from build123d import *

# Parameters (mm, degrees)
SKETCH1_R           = 13.155
BOSS_EXTRUDE1_DEPTH = 10
CHAMFER4_SIZE       = 10


with BuildPart() as part:
    # Sketch1 → Boss-Extrude1 (new body)
    with BuildSketch(Plane(origin=(0, 0, 0), x_dir=(1, 0, 0), z_dir=(0, 1, 0))):
        Polygon((0, 0), (37.5, 64.951905284), (0, 129.903810568), (64.951905284, 92.403810568), (129.903810568, 129.903810568), (92.403810568, 64.951905284), (129.903810568, 0), (64.951905284, 37.5), align=None)
        with Locations(Location((64.951905284, 64.951905284, 0), (0, 0, 270))):
            Circle(SKETCH1_R, mode=Mode.SUBTRACT)
    extrude(amount=BOSS_EXTRUDE1_DEPTH)

    # Chamfer4
    # the kernel refuses this chamfer: 10 mm, written as the material it takes off along each edge
    with BuildSketch(Plane(origin=(64.951905284, 10, -64.951905284), x_dir=(0, 0, 1), z_dir=(-1, 0, 0))) as chamfer4_piece_1:
        Polygon((13.155, -CHAMFER4_SIZE), (13.155 + CHAMFER4_SIZE, 0), (13.155, 0), align=None)
    revolve(axis=Axis((64.951905284, 10, -64.951905284), (0, 1, 0)), mode=Mode.SUBTRACT)
    with BuildSketch(Plane(origin=(-12.85841494, 10, 22.271427981), x_dir=(-0.023812127644090117, -0.9996219169112968, -0.013747938305293196), z_dir=(0.5000000000000011, 0, -0.866025403784438))) as chamfer4_piece_2_section:
        Polygon((CHAMFER4_SIZE * 0.999621916911, -CHAMFER4_SIZE * 0.0274958766106), (-CHAMFER4_SIZE * 0.0274958766106, -CHAMFER4_SIZE * 0.999621916911), (0, 0), align=None)
    chamfer4_piece_2 = extrude(amount=126.433659759, mode=Mode.PRIVATE)
    chamfer4_piece_2 = split(chamfer4_piece_2, bisect_by=Plane(origin=(51.736915966, 6.682227924, -40.292843487), z_dir=(-0.8660254037844383, 0, 0.5000000000000009)), keep=Keep.TOP, mode=Mode.PRIVATE)
    add(chamfer4_piece_2, mode=Mode.SUBTRACT)
    with BuildSketch(Plane(origin=(50.35841494, 10, -42.680477303), x_dir=(-0.02381212764408977, -0.9996219169112968, 0.013747938305292988), z_dir=(-0.5000000000000009, 0, -0.8660254037844383))) as chamfer4_piece_3_section:
        Polygon((CHAMFER4_SIZE * 0.999621916911, -CHAMFER4_SIZE * 0.0274958766106), (-CHAMFER4_SIZE * 0.0274958766106, -CHAMFER4_SIZE * 0.999621916911), (0, 0), align=None)
    chamfer4_piece_3 = extrude(amount=126.433659759, mode=Mode.PRIVATE)
    chamfer4_piece_3 = split(chamfer4_piece_3, bisect_by=Plane(origin=(51.736915966, 6.682227924, -89.610967081), z_dir=(-0.866025403784438, 0, -0.5000000000000011)), keep=Keep.TOP, mode=Mode.PRIVATE)
    add(chamfer4_piece_3, mode=Mode.SUBTRACT)
    with BuildSketch(Plane(origin=(-22.271427981, 10, -142.762225507), x_dir=(0.01374793830529321, -0.9996219169112968, -0.023812127644090134), z_dir=(0.866025403784438, 0, 0.5000000000000012))) as chamfer4_piece_4_section:
        Polygon((CHAMFER4_SIZE * 0.999621916911, -CHAMFER4_SIZE * 0.0274958766106), (-CHAMFER4_SIZE * 0.0274958766106, -CHAMFER4_SIZE * 0.999621916911), (0, 0), align=None)
    chamfer4_piece_4 = extrude(amount=126.433659759, mode=Mode.PRIVATE)
    chamfer4_piece_4 = split(chamfer4_piece_4, bisect_by=Plane(origin=(40.292843487, 6.682227924, -78.166894601), z_dir=(-0.5000000000000012, 0, -0.866025403784438)), keep=Keep.TOP, mode=Mode.PRIVATE)
    add(chamfer4_piece_4, mode=Mode.SUBTRACT)
    with BuildSketch(Plane(origin=(42.680477303, 10, -79.545395628), x_dir=(-0.01374793830529287, -0.9996219169112968, -0.023812127644089548), z_dir=(0.866025403784438, 0, -0.5000000000000012))) as chamfer4_piece_5_section:
        Polygon((CHAMFER4_SIZE * 0.999621916911, -CHAMFER4_SIZE * 0.0274958766106), (-CHAMFER4_SIZE * 0.0274958766106, -CHAMFER4_SIZE * 0.999621916911), (0, 0), align=None)
    chamfer4_piece_5 = extrude(amount=126.433659759, mode=Mode.PRIVATE)
    chamfer4_piece_5 = split(chamfer4_piece_5, bisect_by=Plane(origin=(89.610967081, 6.682227924, -78.166894601), z_dir=(0.5000000000000012, 0, -0.866025403784438)), keep=Keep.TOP, mode=Mode.PRIVATE)
    add(chamfer4_piece_5, mode=Mode.SUBTRACT)
    with BuildSketch(Plane(origin=(142.762225507, 10, -152.175238548), x_dir=(0.023812127644092358, -0.9996219169112965, 0.013747938305294477), z_dir=(-0.5000000000000007, 0, 0.8660254037844384))) as chamfer4_piece_6_section:
        Polygon((CHAMFER4_SIZE * 0.999621916911, -CHAMFER4_SIZE * 0.0274958766106), (-CHAMFER4_SIZE * 0.0274958766106, -CHAMFER4_SIZE * 0.999621916911), (0, 0), align=None)
    chamfer4_piece_6 = extrude(amount=126.433659759, mode=Mode.PRIVATE)
    chamfer4_piece_6 = split(chamfer4_piece_6, bisect_by=Plane(origin=(78.166894601, 6.682227924, -89.610967081), z_dir=(0.8660254037844382, 0, -0.500000000000001)), keep=Keep.TOP, mode=Mode.PRIVATE)
    add(chamfer4_piece_6, mode=Mode.SUBTRACT)
    with BuildSketch(Plane(origin=(79.545395628, 10, -87.223333264), x_dir=(0.023812127644090287, -0.9996219169112968, -0.013747938305293292), z_dir=(0.500000000000001, 0, 0.8660254037844382))) as chamfer4_piece_7_section:
        Polygon((CHAMFER4_SIZE * 0.999621916911, -CHAMFER4_SIZE * 0.0274958766106), (-CHAMFER4_SIZE * 0.0274958766106, -CHAMFER4_SIZE * 0.999621916911), (0, 0), align=None)
    chamfer4_piece_7 = extrude(amount=126.433659759, mode=Mode.PRIVATE)
    chamfer4_piece_7 = split(chamfer4_piece_7, bisect_by=Plane(origin=(78.166894601, 6.682227924, -40.292843487), z_dir=(0.8660254037844384, 0, 0.5000000000000007)), keep=Keep.TOP, mode=Mode.PRIVATE)
    add(chamfer4_piece_7, mode=Mode.SUBTRACT)
    with BuildSketch(Plane(origin=(152.175238548, 10, 12.85841494), x_dir=(-0.013747938305293, -0.9996219169112968, 0.023812127644089767), z_dir=(-0.8660254037844379, 0, -0.5000000000000012))) as chamfer4_piece_8_section:
        Polygon((CHAMFER4_SIZE * 0.999621916911, -CHAMFER4_SIZE * 0.0274958766106), (-CHAMFER4_SIZE * 0.0274958766106, -CHAMFER4_SIZE * 0.999621916911), (0, 0), align=None)
    chamfer4_piece_8 = extrude(amount=126.433659759, mode=Mode.PRIVATE)
    chamfer4_piece_8 = split(chamfer4_piece_8, bisect_by=Plane(origin=(89.610967081, 6.682227924, -51.736915966), z_dir=(0.5000000000000012, 0, 0.8660254037844379)), keep=Keep.TOP, mode=Mode.PRIVATE)
    add(chamfer4_piece_8, mode=Mode.SUBTRACT)
    with BuildSketch(Plane(origin=(87.223333264, 10, -50.35841494), x_dir=(0.013747938305293599, -0.9996219169112968, 0.0238121276440908), z_dir=(-0.8660254037844379, 0, 0.5000000000000012))) as chamfer4_piece_9_section:
        Polygon((CHAMFER4_SIZE * 0.999621916911, -CHAMFER4_SIZE * 0.0274958766106), (-CHAMFER4_SIZE * 0.0274958766106, -CHAMFER4_SIZE * 0.999621916911), (0, 0), align=None)
    chamfer4_piece_9 = extrude(amount=126.433659759, mode=Mode.PRIVATE)
    chamfer4_piece_9 = split(chamfer4_piece_9, bisect_by=Plane(origin=(40.292843487, 6.682227924, -51.736915966), z_dir=(-0.5000000000000012, 0, 0.8660254037844379)), keep=Keep.TOP, mode=Mode.PRIVATE)
    add(chamfer4_piece_9, mode=Mode.SUBTRACT)
    with BuildSketch(Plane(origin=(-12.85841494, 10, 22.271427981), x_dir=(-0.023812127644090117, -0.9996219169112968, -0.013747938305293196), z_dir=(0.5000000000000011, 0, -0.866025403784438))) as chamfer4_piece_10a_section:
        Polygon((CHAMFER4_SIZE * 0.999621916911, -CHAMFER4_SIZE * 0.0274958766106), (-CHAMFER4_SIZE * 0.0274958766106, -CHAMFER4_SIZE * 0.999621916911), (0, 0), align=None)
    chamfer4_piece_10a = extrude(amount=126.433659759, mode=Mode.PRIVATE)
    chamfer4_piece_10a = split(chamfer4_piece_10a, bisect_by=Plane(origin=(36.018509, 6.773025627, -67.517922967), z_dir=(0.8660254037844383, 0, -0.5000000000000009)), keep=Keep.TOP, mode=Mode.PRIVATE)
    with BuildSketch(Plane(origin=(50.35841494, 10, -42.680477303), x_dir=(-0.02381212764408977, -0.9996219169112968, 0.013747938305292988), z_dir=(-0.5000000000000009, 0, -0.8660254037844383))) as chamfer4_piece_10b_section:
        Polygon((CHAMFER4_SIZE * 0.999621916911, -CHAMFER4_SIZE * 0.0274958766106), (-CHAMFER4_SIZE * 0.0274958766106, -CHAMFER4_SIZE * 0.999621916911), (0, 0), align=None)
    chamfer4_piece_10b = extrude(amount=126.433659759, mode=Mode.PRIVATE)
    chamfer4_piece_10b = split(chamfer4_piece_10b, bisect_by=Plane(origin=(36.018509, 6.773025627, -62.385887601), z_dir=(0.866025403784438, 0, 0.5000000000000011)), keep=Keep.TOP, mode=Mode.PRIVATE)
    chamfer4_piece_10 = chamfer4_piece_10a & chamfer4_piece_10b
    add(chamfer4_piece_10, mode=Mode.SUBTRACT)
    with BuildSketch(Plane(origin=(-22.271427981, 10, -142.762225507), x_dir=(0.01374793830529321, -0.9996219169112968, -0.023812127644090134), z_dir=(0.866025403784438, 0, 0.5000000000000012))) as chamfer4_piece_11a_section:
        Polygon((CHAMFER4_SIZE * 0.999621916911, -CHAMFER4_SIZE * 0.0274958766106), (-CHAMFER4_SIZE * 0.0274958766106, -CHAMFER4_SIZE * 0.999621916911), (0, 0), align=None)
    chamfer4_piece_11a = extrude(amount=126.433659759, mode=Mode.PRIVATE)
    chamfer4_piece_11a = split(chamfer4_piece_11a, bisect_by=Plane(origin=(67.517922967, 6.773025627, -93.885301568), z_dir=(0.5000000000000012, 0, 0.866025403784438)), keep=Keep.TOP, mode=Mode.PRIVATE)
    with BuildSketch(Plane(origin=(42.680477303, 10, -79.545395628), x_dir=(-0.01374793830529287, -0.9996219169112968, -0.023812127644089548), z_dir=(0.866025403784438, 0, -0.5000000000000012))) as chamfer4_piece_11b_section:
        Polygon((CHAMFER4_SIZE * 0.999621916911, -CHAMFER4_SIZE * 0.0274958766106), (-CHAMFER4_SIZE * 0.0274958766106, -CHAMFER4_SIZE * 0.999621916911), (0, 0), align=None)
    chamfer4_piece_11b = extrude(amount=126.433659759, mode=Mode.PRIVATE)
    chamfer4_piece_11b = split(chamfer4_piece_11b, bisect_by=Plane(origin=(62.385887601, 6.773025627, -93.885301568), z_dir=(-0.5000000000000012, 0, 0.866025403784438)), keep=Keep.TOP, mode=Mode.PRIVATE)
    chamfer4_piece_11 = chamfer4_piece_11a & chamfer4_piece_11b
    add(chamfer4_piece_11, mode=Mode.SUBTRACT)
    with BuildSketch(Plane(origin=(142.762225507, 10, -152.175238548), x_dir=(0.023812127644092358, -0.9996219169112965, 0.013747938305294477), z_dir=(-0.5000000000000007, 0, 0.8660254037844384))) as chamfer4_piece_12a_section:
        Polygon((CHAMFER4_SIZE * 0.999621916911, -CHAMFER4_SIZE * 0.0274958766106), (-CHAMFER4_SIZE * 0.0274958766106, -CHAMFER4_SIZE * 0.999621916911), (0, 0), align=None)
    chamfer4_piece_12a = extrude(amount=126.433659759, mode=Mode.PRIVATE)
    chamfer4_piece_12a = split(chamfer4_piece_12a, bisect_by=Plane(origin=(93.885301568, 6.773025627, -62.385887601), z_dir=(-0.8660254037844382, 0, 0.500000000000001)), keep=Keep.TOP, mode=Mode.PRIVATE)
    with BuildSketch(Plane(origin=(79.545395628, 10, -87.223333264), x_dir=(0.023812127644090287, -0.9996219169112968, -0.013747938305293292), z_dir=(0.500000000000001, 0, 0.8660254037844382))) as chamfer4_piece_12b_section:
        Polygon((CHAMFER4_SIZE * 0.999621916911, -CHAMFER4_SIZE * 0.0274958766106), (-CHAMFER4_SIZE * 0.0274958766106, -CHAMFER4_SIZE * 0.999621916911), (0, 0), align=None)
    chamfer4_piece_12b = extrude(amount=126.433659759, mode=Mode.PRIVATE)
    chamfer4_piece_12b = split(chamfer4_piece_12b, bisect_by=Plane(origin=(93.885301568, 6.773025627, -67.517922967), z_dir=(-0.8660254037844384, 0, -0.5000000000000007)), keep=Keep.TOP, mode=Mode.PRIVATE)
    chamfer4_piece_12 = chamfer4_piece_12a & chamfer4_piece_12b
    add(chamfer4_piece_12, mode=Mode.SUBTRACT)
    with BuildSketch(Plane(origin=(152.175238548, 10, 12.85841494), x_dir=(-0.013747938305293, -0.9996219169112968, 0.023812127644089767), z_dir=(-0.8660254037844379, 0, -0.5000000000000012))) as chamfer4_piece_13a_section:
        Polygon((CHAMFER4_SIZE * 0.999621916911, -CHAMFER4_SIZE * 0.0274958766106), (-CHAMFER4_SIZE * 0.0274958766106, -CHAMFER4_SIZE * 0.999621916911), (0, 0), align=None)
    chamfer4_piece_13a = extrude(amount=126.433659759, mode=Mode.PRIVATE)
    chamfer4_piece_13a = split(chamfer4_piece_13a, bisect_by=Plane(origin=(62.385887601, 6.773025627, -36.018509), z_dir=(-0.5000000000000012, 0, -0.8660254037844379)), keep=Keep.TOP, mode=Mode.PRIVATE)
    with BuildSketch(Plane(origin=(87.223333264, 10, -50.35841494), x_dir=(0.013747938305293599, -0.9996219169112968, 0.0238121276440908), z_dir=(-0.8660254037844379, 0, 0.5000000000000012))) as chamfer4_piece_13b_section:
        Polygon((CHAMFER4_SIZE * 0.999621916911, -CHAMFER4_SIZE * 0.0274958766106), (-CHAMFER4_SIZE * 0.0274958766106, -CHAMFER4_SIZE * 0.999621916911), (0, 0), align=None)
    chamfer4_piece_13b = extrude(amount=126.433659759, mode=Mode.PRIVATE)
    chamfer4_piece_13b = split(chamfer4_piece_13b, bisect_by=Plane(origin=(67.517922967, 6.773025627, -36.018509), z_dir=(0.5000000000000012, 0, -0.8660254037844379)), keep=Keep.TOP, mode=Mode.PRIVATE)
    chamfer4_piece_13 = chamfer4_piece_13a & chamfer4_piece_13b
    add(chamfer4_piece_13, mode=Mode.SUBTRACT)


solid = part.part
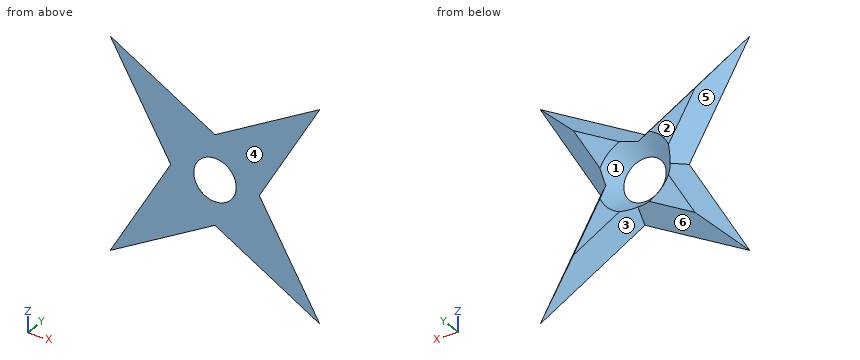
Design review of the part built by this model. Coordinates are the model's own, in mm. Face numbers are marked on the shaded views. A direction names the side the tool comes from. Coordinates: 2 decimals unless noted, no trailing zeros. Loops run counter-clockwise (first coordinate to the right, second up) from the corner with the lowest first, then second, coordinate; pieces in that order, holes last. Notation, with made-up numbers: (40.25, -18.5) -> (98.25, -18.5) arc R28 ccw to (98.25, 20.5) -> close; hole circle Ø8 at (88.25, -33). An arc over 180 degrees is marked (long way). Use a Markdown table: item, result. Add a question column.
Item 1: Clearance check with flat-ended pins moving along their axes: P1, Ø3, axis at x = 58.5, y = 8.5, coming from the -Z side; P2, Ø1, axis at x = 55.5, y = 2.5, coming from the +Z side; P3, Ø1, axis at y = 7, z = -26, coming from the +X side. State where each tip first meets the part, or that it passes through.
Item 2: We need section A-A, the plane y = 8.25. Write out the cut boundary in (x, z) (3 decimals).
Item 3: We need section C-C, the plane x = 97. Write out the cut boundary in (y, z), and give its area (3 significant figures).
Item 4: Wall thickness on L1, parallel to Z at x = 95.5, y = 8; L2, parallel to X at y = 2.25, z = -68; L3, parallel to X at y = 7.75, z = -41: over which ranges is each line inside the solid? List them lowest first. Write a range as from..to.
Item 5: We need section D-D, the plane z = -23. Write out the cut boundary in (x, y), and give its area (3 significant figures).
Item 6: Machinability: for the marked faces 4, 5 and 6, which of the approach directions +Z, -Z, +X, -X, +Y, -Y give a long, thin tool a straight path to every point of the face, cutting with its end or side? Answer none if there is none.
Item 7: The part is to be moulded in two halves that separate along Z. For the marked faces 1, 2 and 3, say which applies: +Z half, -Z half, draft (parallel to the pull), parting line (faces both ways), or undercut.
Item 8: We need section B-B, the plane z = -119. Write out the cut boundary in (x, y), and give its area (4 significant figures).
Numbers:
| question | item | result |
|---|---|---|
| 1 | P1 | stops at z = -88.25 |
| 1 | P2 | stops at z = -34.28 |
| 1 | P3 | stops at x = 107.46 |
| 2 | outline | (22.539, -107.364) -> (59.951, -85.765) arc R21.405 cw to (44.139, -69.952) -> close; (22.539, -22.539) -> (44.139, -59.951) arc R21.405 cw to (59.951, -44.139) -> close; (69.952, -85.765) -> (107.364, -107.364) -> (85.765, -69.952) arc R21.405 cw to start; (69.952, -44.139) arc R21.405 cw to (85.765, -59.951) -> (107.364, -22.539) -> close |
| 3 | outline | (0, -110.91) -> (10, -99.36) -> (10, -92.91) -> (0, -72.91) -> close; (0, -56.99) -> (10, -36.99) -> (10, -30.54) -> (0, -19) -> close |
| 3 | area | 444 mm^2 |
| 4 | L1 | z = -100.8..-86.31, -43.59..-29.1 |
| 4 | L2 | x = 38.34..49.85, 80.05..91.57 |
| 4 | L3 | x = 32.62..55.51, 74.39..97.28 |
| 5 | outline | (13.28, 0) -> (39.84, 0) -> (23, 8.42) -> close; (90.07, 0) -> (116.62, 0) -> (106.9, 8.42) -> close |
| 5 | area | 224 mm^2 |
| 6 | face 4 | +Z, -Z, +X, -X, -Y |
| 6 | face 5 | -X, +Y |
| 6 | face 6 | -Z, +Y |
| 7 | face 1 | undercut |
| 7 | face 2 | draft |
| 7 | face 3 | -Z half |
| 8 | outline | (6.3, 0) -> (18.89, 0) -> (10.9, 3.99) -> close; (111.02, 0) -> (123.61, 0) -> (119, 3.99) -> close |
| 8 | area | 50.25 mm^2 |
